from build123d import *

# Parameters (mm, degrees)
SKETCH1_W               = 11
SKETCH1_H               = 31
BOSS_EXTRUDE1_DEPTH     = 3.81
SKETCH1_W_2             = 31
SKETCH1_H_2             = 11
BOSS_EXTRUDE1_2_DEPTH   = 3.81
BOSS_EXTRUDE1_3_DEPTH   = 3.81
BOSS_EXTRUDE1_4_DEPTH   = 3.81
BOSS_EXTRUDE1_5_DEPTH   = 3.81
SKETCH1_W_3             = 80
SKETCH1_H_3             = 100
SKETCH1_W_4             = 78.5
SKETCH1_H_4             = 98.5
BOSS_EXTRUDE1_6_DEPTH   = 3.81
SKETCH3_W               = 80
SKETCH3_H               = 100
SKETCH3_W_2             = 31
SKETCH3_H_2             = 11
SKETCH3_W_3             = 11
SKETCH3_H_3             = 31
BOSS_EXTRUDE2_DEPTH     = 1.5875
FILLET1_R               = 0.05
SKETCH4_W               = 80
SKETCH4_H               = 100
BOSS_EXTRUDE3_DEPTH     = 6.191
CUT_EXTRUDE1_DEPTH      = 65.807561295
CUT_EXTRUDE1_DEPTH_BACK = 65.807561295
SKETCH5_W               = 56.628696971
SKETCH5_H               = 106.323278981
CUT_EXTRUDE2_DEPTH      = 3.81
SKETCH7_W               = 1.5875
SKETCH7_H               = 11
BOSS_EXTRUDE4_DEPTH     = 0.75
SKETCH8_W               = 11.5885
SKETCH8_H               = 100
BOSS_EXTRUDE5_DEPTH     = 1


with BuildPart() as part:
    # Sketch1 → Boss-Extrude1 (new body)
    with BuildSketch(Plane.XY):
        Polygon((-26.313903431, 0.439060111), (-31.5, 2.5), (-31.5, 35.5), (-25.083245041, 38.05), (-18.5, 35.5), (-18.5, 2.5), (-23.846750882, 0.428952262), (-23.616775358, 0.03062297), (-23.846750882, -0.367706323), (-18.5, -2.438754061), (-18.5, -35.438754061), (-25.083245041, -37.988754061), (-31.5, -35.438754061), (-31.5, -2.438754061), (-26.313903431, -0.377814172), (-26.549714725, 0.03062297), align=None)
        with Locations((-25, -18.938754061)):
            Rectangle(SKETCH1_W, SKETCH1_H, mode=Mode.SUBTRACT)
        with Locations((-25, 19)):
            Rectangle(SKETCH1_W, SKETCH1_H, mode=Mode.SUBTRACT)
    extrude(amount=BOSS_EXTRUDE1_DEPTH)



with BuildPart() as body_2:
    # Sketch1 → Boss-Extrude1 2 (new body)
    with BuildSketch(Plane.XY):
        Polygon((-19.05, 0.03062297), (-16.5, 6.5), (16.5, 6.5), (19.05, 0.03062297), (16.5, -6.438754061), (-16.5, -6.438754061), align=None)
        Rectangle(SKETCH1_W_2, SKETCH1_H_2, mode=Mode.SUBTRACT)
    extrude(amount=BOSS_EXTRUDE1_2_DEPTH)


with BuildPart() as body_3:
    # Sketch1 → Boss-Extrude1 3 (new body)
    with BuildSketch(Plane.XY):
        Polygon((26.313903431, 0.439060111), (26.549714725, 0.03062297), (26.313903431, -0.377814172), (31.5, -2.438754061), (31.5, -35.438754061), (25.083245041, -37.988754061), (18.5, -35.438754061), (18.5, -2.438754061), (23.846750882, -0.367706323), (23.616775358, 0.03062297), (23.846750882, 0.428952262), (18.5, 2.5), (18.5, 35.5), (25.083245041, 38.05), (31.5, 35.5), (31.5, 2.5), align=None)
        with Locations((25, 19)):
            Rectangle(SKETCH1_W, SKETCH1_H, mode=Mode.SUBTRACT)
        with Locations((25, -18.938754061)):
            Rectangle(SKETCH1_W, SKETCH1_H, mode=Mode.SUBTRACT)
    extrude(amount=BOSS_EXTRUDE1_3_DEPTH)


with BuildPart() as body_4:
    # Sketch1 → Boss-Extrude1 4 (new body)
    with BuildSketch(Plane.XY):
        Polygon((-16.5, 31.52602227), (-19.05, 38.013011135), (-16.5, 44.5), (16.5, 44.5), (19.05, 38.013011135), (16.5, 31.52602227), align=None)
        with Locations((0, 38)):
            Rectangle(SKETCH1_W_2, SKETCH1_H_2, mode=Mode.SUBTRACT)
    extrude(amount=BOSS_EXTRUDE1_4_DEPTH)


with BuildPart() as body_5:
    # Sketch1 → Boss-Extrude1 5 (new body)
    with BuildSketch(Plane.XY):
        Polygon((16.5, -31.464776331), (19.05, -37.951765196), (16.5, -44.438754061), (-16.5, -44.438754061), (-19.05, -37.951765196), (-16.5, -31.464776331), align=None)
        with Locations((0, -37.938754061)):
            Rectangle(SKETCH1_W_2, SKETCH1_H_2, mode=Mode.SUBTRACT)
    extrude(amount=BOSS_EXTRUDE1_5_DEPTH)


with BuildPart() as body_6:
    # Sketch1 → Boss-Extrude1 6 (new body)
    with BuildSketch(Plane.XY):
        Rectangle(SKETCH1_W_3, SKETCH1_H_3)
        Rectangle(SKETCH1_W_4, SKETCH1_H_4, mode=Mode.SUBTRACT)
    extrude(amount=BOSS_EXTRUDE1_6_DEPTH)


with BuildPart() as part_1:
    add(part.part)

    add(body_2.part)  # Boss-Extrude2 merges body 2

    add(body_3.part)  # Boss-Extrude2 merges body 3

    add(body_4.part)  # Boss-Extrude2 merges body 4

    add(body_5.part)  # Boss-Extrude2 merges body 5

    add(body_6.part)  # Boss-Extrude2 merges body 6
    # Sketch3 → Boss-Extrude2 (add)
    with BuildSketch(Plane.XY.offset(3.81)):
        Rectangle(SKETCH3_W, SKETCH3_H)
        with Locations((0, -37.938754061)):
            Rectangle(SKETCH3_W_2, SKETCH3_H_2, mode=Mode.SUBTRACT)
        Rectangle(SKETCH3_W_2, SKETCH3_H_2, mode=Mode.SUBTRACT)
        with Locations((-25, -18.938754061)):
            Rectangle(SKETCH3_W_3, SKETCH3_H_3, mode=Mode.SUBTRACT)
        with Locations((-25, 19)):
            Rectangle(SKETCH3_W_3, SKETCH3_H_3, mode=Mode.SUBTRACT)
        with Locations((0, 38)):
            Rectangle(SKETCH3_W_2, SKETCH3_H_2, mode=Mode.SUBTRACT)
        with Locations((25, 19)):
            Rectangle(SKETCH3_W_3, SKETCH3_H_3, mode=Mode.SUBTRACT)
        with Locations((25, -18.938754061)):
            Rectangle(SKETCH3_W_3, SKETCH3_H_3, mode=Mode.SUBTRACT)
    extrude(amount=BOSS_EXTRUDE2_DEPTH)

    # Fillet1
    fillet1_edges = [part_1.edges().sort_by_distance(p)[0] for p in [
        (39.25, 49.25, 1.905),
        (39.25, -49.25, 1.905),
        (-39.25, -49.25, 1.905),
        (-39.25, 49.25, 1.905),
    ]]
    fillet(fillet1_edges, radius=FILLET1_R)

    # Sketch4 → Boss-Extrude3 (add)
    with BuildSketch(Plane(origin=(0, 0, 0), x_dir=(-1, 0, 0), z_dir=(0, 0, -1))):
        Rectangle(SKETCH4_W, SKETCH4_H)
        with BuildLine():
            Line((-39.2, -49.25), (39.2, -49.25))
            ThreePointArc((39.2, -49.25), (39.235355339, -49.235355339), (39.25, -49.2))
            Line((39.25, -49.2), (39.25, 49.2))
            ThreePointArc((39.25, 49.2), (39.235355339, 49.235355339), (39.2, 49.25))
            Line((39.2, 49.25), (-39.2, 49.25))
            ThreePointArc((-39.2, 49.25), (-39.235355339, 49.235355339), (-39.25, 49.2))
            Line((-39.25, 49.2), (-39.25, -49.2))
            ThreePointArc((-39.25, -49.2), (-39.235355339, -49.235355339), (-39.2, -49.25))
        make_face(mode=Mode.SUBTRACT)
    extrude(amount=BOSS_EXTRUDE3_DEPTH)

    # Sketch5 → Cut-Extrude1 (cut, two sides: drawn at the far end of the back side and taken through both)
    with BuildSketch(Plane(origin=(0, 0, 3.81), x_dir=(-1, 0, 0), z_dir=(0, 0, -1)).offset(-CUT_EXTRUDE1_DEPTH_BACK)):
        with Locations((13.564348486, -0.302353259)):
            Rectangle(SKETCH5_W, SKETCH5_H)
    extrude(amount=CUT_EXTRUDE1_DEPTH + CUT_EXTRUDE1_DEPTH_BACK, mode=Mode.SUBTRACT)

    # Sketch6 → Cut-Extrude2 (cut)
    with BuildSketch(Plane(origin=(0, 0, 0), x_dir=(-1, 0, 0), z_dir=(0, 0, -1))):
        Polygon((-16.5, -44.438754061), (-14.75, -44.438754061), (-14.75, -43.438754061), (-15.5, -43.438754061), (-15.5, -32.438754061), (-14.75, -32.438754061), (-14.75, -31.464776331), (-16.5, -31.464776331), (-19.05, -37.951765196), align=None)
        Polygon((-16.5, -6.438754061), (-14.75, -6.438754061), (-14.75, -5.5), (-15.5, -5.5), (-15.5, 5.5), (-14.75, 5.5), (-14.75, 6.5), (-16.5, 6.5), (-19.05, 0.03062297), align=None)
        Polygon((-16.5, 31.52602227), (-14.75, 31.52602227), (-14.75, 32.5), (-15.5, 32.5), (-15.5, 43.5), (-14.75, 43.5), (-14.75, 44.5), (-16.5, 44.5), (-19.05, 38.013011135), align=None)
    extrude(amount=-CUT_EXTRUDE2_DEPTH, mode=Mode.SUBTRACT)

    # Sketch7 → Boss-Extrude4 (add)
    with BuildSketch(Plane.ZY.offset(-15.5)):
        with Locations((4.60375, 38)):
            Rectangle(SKETCH7_W, SKETCH7_H)
        with Locations((4.60375, 0)):
            Rectangle(SKETCH7_W, SKETCH7_H)
        with Locations((4.60375, -37.938754061)):
            Rectangle(SKETCH7_W, SKETCH7_H)
    extrude(amount=BOSS_EXTRUDE4_DEPTH)

    # Sketch8 → Boss-Extrude5 (add)
    with BuildSketch(Plane.ZY.offset(-14.75)):
        with Locations((-0.39675, 0)):
            Rectangle(SKETCH8_W, SKETCH8_H)
    extrude(amount=-BOSS_EXTRUDE5_DEPTH)


solid = part_1.part
Here's how the part is built. I have some questions about the finished solid (model axes, mm). A direction names the side the tool comes from. Coordinates: 2 decimals unless noted, no trailing zeros. Order: outer loops, then holes, each group sorted by start corner. A loop starts at its lowest first (then second) coordinate and runs counter-clockwise, first axis right, second up. Notation, with made-up numbers: (56.5, 39.5) -> (90.5, 39.5) arc R15 ccw to (90.5, 61.5) -> close; hole circle Ø7 at (-27, 64.25). An arc over 180 degrees is marked (long way). Answer in a Markdown table with one row per item.
(1) Please list where these lines run through material, in increasing order: probe 1 along X at (y, z) = (-31.5, 3); probe 2 along Y at (x, z) = (33.25, 0); probe 3 along X at (y, z) = (45.5, 0.75).
Answer key:
| item | result |
|---|---|
| probe 1 | 14.75 to 15.75, 18.5 to 19.5, 30.5 to 31.5, 39.25 to 40 |
| probe 2 | -50 to -49.25, 49.25 to 50 |
| probe 3 | 14.75 to 15.75, 39.25 to 40 |
(2) I want a section at B-B on z = -3. List the corners of the cut face in (x, y) for me.
Answer key:
| item | result |
|---|---|
| outline | (14.75, -50) -> (40, -50) -> (40, 50) -> (14.75, 50) -> close; hole (15.75, -49.25) -> (39.2, -49.25) arc R0.05 ccw to (39.25, -49.2) -> (39.25, 49.2) arc R0.05 ccw to (39.2, 49.25) -> (15.75, 49.25) -> close |
(3) I want a section at D-D on y = 39.5. List the corners of the cut face in (x, z) for me, then the cut area to 3 significant figures.
Answer key:
| item | result |
|---|---|
| outline | (14.75, -6.19) -> (15.75, -6.19) -> (15.75, 3.81) -> (39.25, 3.81) -> (39.25, -6.19) -> (40, -6.19) -> (40, 5.4) -> (14.75, 5.4) -> close |
| area | 57.6 mm^2 |
(4) I want a section at C-C on x = 38. List the corners of the cut face in (y, z) for me, then the cut area to 3 significant figures.
Answer key:
| item | result |
|---|---|
| outline | (-50, -6.19) -> (-49.25, -6.19) -> (-49.25, 3.81) -> (49.25, 3.81) -> (49.25, -6.19) -> (50, -6.19) -> (50, 5.4) -> (-50, 5.4) -> close |
| area | 174 mm^2 |
(5) On a 3-axis mill with a long thin cutter (end or side, diameter ignored), from which of +Z, -Z, +X, -X, +Y, -Y can I reach the whole of each face in a straight line? I mean faces 1 (the face through (25, -34.439, 3)), 2 (the face through (28.337, -36.696, 1.878)). Say none if no direction works.
Answer key:
| item | result |
|---|---|
| face 1 | +Z, -Z |
| face 2 | -Z |
(6) I want a section at A-A on y = 25.5. List the corners of the cut face in (x, z) for me.
Answer key:
| item | result |
|---|---|
| outline | (14.75, -6.19) -> (15.75, -6.19) -> (15.75, 3.81) -> (18.5, 3.81) -> (18.5, 0) -> (19.5, 0) -> (19.5, 5.4) -> (14.75, 5.4) -> close; (30.5, 0) -> (31.5, 0) -> (31.5, 3.81) -> (39.25, 3.81) -> (39.25, -6.19) -> (40, -6.19) -> (40, 5.4) -> (30.5, 5.4) -> close |
(7) Will these pins go through, and if not, where does the flat tip stop? pin 1 Ø2 at (x, y) = (22, -3.5) entering from -Z; pin 2 Ø1.5 at (x, y) = (21.5, -40) entering from -Z.
Answer key:
| item | result |
|---|---|
| pin 1 | z = 0 |
| pin 2 | z = 3.81 |
(8) Thinking about a two-plate mould opening in X: for faces 3 (the face through (25, -3.439, 3)), 4 (the face through (15, 0, -6.191)), 5 (the face through (14.75, 1, 0)), which applies, +X half, -X half, draft (parallel to the pull), parting line (faces both ways), or undercut?
Answer key:
| item | result |
|---|---|
| face 3 | undercut |
| face 4 | draft |
| face 5 | -X half |
